from build123d import *

# Parameters (mm, degrees)
SKETCH_1_W              = 16
SKETCH_1_H              = 3
EXTRUDE_1_DEPTH         = 10
SKETCH_2_W              = 30
SKETCH_2_H              = 20
EXTRUDE_2_DEPTH         = 3
HOLE_WIZARD_2_2_2_2_1_D = 2.2
HOLE_WIZARD_2_2_2_2_2_D = 2.2
FILLET_1_R              = 0.7


with BuildPart() as part:
    # 草图1 → 凸台-拉伸1 (new body)
    with BuildSketch(Plane.XY):
        with Locations((0, 1.5)):
            Rectangle(SKETCH_1_W, SKETCH_1_H)
    extrude(amount=-EXTRUDE_1_DEPTH)

    # 草图2 → 凸台-拉伸2 (add)
    with BuildSketch(Plane.XY):
        with Locations((-7, 10)):
            Rectangle(SKETCH_2_W, SKETCH_2_H)
    extrude(amount=EXTRUDE_2_DEPTH)

    # Ø2.2 (2.2) 直径孔1 (through all)
    with Locations(Plane(origin=(0, 3, 0), x_dir=(1, 0, 0), z_dir=(0, 1, 0))):
        with Locations((-5, 5), (5, 5)):
            Hole(HOLE_WIZARD_2_2_2_2_1_D / 2)

    # Ø2.2 (2.2) 直径孔2 (through all)
    with Locations(Plane.XY.offset(3)):
        with Locations((-17, 12.52), (-7, 12.52), (3, 12.52)):
            Hole(HOLE_WIZARD_2_2_2_2_2_D / 2)

    # 圆角1
    fillet_1_edges = [part.edges().sort_by_distance(p)[0] for p in [
        (8, 1.5, -10),
        (8, 11.5, 0),
        (-7, 20, 0),
        (8, 20, 1.5),
        (-22, 10, 0),
        (-22, 20, 1.5),
        (-15, 0, 0),
        (-22, 0, 1.5),
        (8, 10, 3),
        (-7, 20, 3),
        (0, 3, -10),
        (-22, 10, 3),
        (-7, 0, 3),
        (-8, 1.5, -10),
        (0, 3, 0),
        (-8, 1.5, 0),
        (-8, 3, -5),
        (8, 3, -5),
        (8, 0, -3.5),
        (-8, 0, -5),
        (0, 0, -10),
    ]]
    fillet(fillet_1_edges, radius=FILLET_1_R)


solid = part.part
Could you check a few things on this model? Use its own coordinates, in mm. A direction names the side the tool comes from. Give positions to 0.01 mm unless a question says otherwise; leave off trailing zeros. Order: outer loops, then holes, each group sorted by start corner. A loop starts at its lowest first (then second) coordinate and runs counter-clockwise, first axis right, second up. Notation, with made-up numbers: (-14.5, 5) -> (44.5, 5) arc R23 ccw to (44.5, 25) -> close; hole circle Ø11 at (68, 34.5). An arc over 180 degrees is marked (long way). Return JSON: item names as keys, results as strings.
1. On a 3-axis mill with a long thin cutter (end or side, diameter ignored), from which of +Z, -Z, +X, -X, +Y, -Y can I reach the whole of each face in a straight line? I mean faces 1 (the flat face through (-8, 1, -5)), 2 (the flat face through (0, 3, -5)), 3 (the flat face through (8, 7, 1)). Say none if no direction works.
Answer list:
{"face 1": "-Z, -X, +Y, -Y", "face 2": "-Z, +X, -X, +Y", "face 3": "+Z, -Z, +X, +Y, -Y"}
2. For pin 1 Ø9.5 at (x, y) = (-9, 9.5) entering from -Z; pin 2 Ø1.3 at (y, z) = (1.5, -4) entering from -X; pin 3 Ø6 at (x, z) = (-12.5, -8) entering from +Y; pin 4 Ø2.5 at (x, z) = (5, -5) entering from +Y, each with a flat end and sliding along its axis, tell me the tip position at first contact or that it passes through.
Answer list:
{"pin 1": "stops at z = 0", "pin 2": "stops at x = -8", "pin 3": "passes through", "pin 4": "stops at y = 3"}
3. Imagine slicing it at A-A on x = -17. List the corners of the cut face in (y, z) for me, then the cut area to 3 significant figures.
Answer list:
{"outline": "(0, 0.7) arc R0.7 ccw to (0.7, 0) -> (11.42, 0) -> (11.42, 3) -> (0.7, 3) arc R0.7 ccw to (0, 2.3) -> close; (13.62, 0) -> (19.3, 0) arc R0.7 ccw to (20, 0.7) -> (20, 2.3) arc R0.7 ccw to (19.3, 3) -> (13.62, 3) -> close", "area": "53.0 mm2"}
4. I need wall thicknesses on line 1 (X direction, y = 1.75, z = -5); line 2 (Y direction, x = -17, z = 1); line 3 (Z direction, x = 6, y = 8). Which ranges of each line are inside material? Lowest first, please. Write a range as from..to.
Answer list:
{"line 1": "x = -8..-6.1, -3.9..3.9, 6.1..8", "line 2": "y = 0..11.42, 13.62..20", "line 3": "z = 0..3"}
5. Imagine slicing it at D-D on z = -5. List the corners of the cut face in (x, y) for me, then the cut area to 3 significant figures.
Answer list:
{"outline": "(-8, 0.7) arc R0.7 ccw to (-7.3, 0) -> (-6.1, 0) -> (-6.1, 3) -> (-7.3, 3) arc R0.7 ccw to (-8, 2.3) -> close; (-3.9, 0) -> (3.9, 0) -> (3.9, 3) -> (-3.9, 3) -> close; (6.1, 0) -> (7.3, 0) arc R0.7 ccw to (8, 0.7) -> (8, 2.3) arc R0.7 ccw to (7.3, 3) -> (6.1, 3) -> close", "area": "34.4 mm2"}
6. Imagine slicing it at B-B on z = 1.5. List the corners of the cut face in (x, y) for me.
Answer list:
{"outline": "(-22, 0.7) arc R0.7 ccw to (-21.3, 0) -> (7.3, 0) arc R0.7 ccw to (8, 0.7) -> (8, 19.3) arc R0.7 ccw to (7.3, 20) -> (-21.3, 20) arc R0.7 ccw to (-22, 19.3) -> close; hole circle Ø2.2 at (-17, 12.52); hole circle Ø2.2 at (-7, 12.52); hole circle Ø2.2 at (3, 12.52)"}
7. Imagine slicing it at C-C on y = 15. List the corners of the cut face in (x, z) for me.
Answer list:
{"outline": "(-22, 0.7) arc R0.7 ccw to (-21.3, 0) -> (7.3, 0) arc R0.7 ccw to (8, 0.7) -> (8, 2.3) arc R0.7 ccw to (7.3, 3) -> (-21.3, 3) arc R0.7 ccw to (-22, 2.3) -> close"}
8. Thinking about a two-plate mould opening in Z: for faces 4 (the cylindrical face through (-4.189, 1.479, -5.743)), 5 (the cylindrical face through (-16.189, 13.263, 1.479)), 6 (the flat face through (-7, 10, 3)), 7 (the cylindrical face through (4.41, 1.48, -5.93)), which applies, pulls with the +Z half, pulls with the -Z half, needs draft (parallel to the pull), parting line crosses it, or undercut?
Answer list:
{"face 4": "undercut", "face 5": "needs draft", "face 6": "pulls with the +Z half", "face 7": "undercut"}
